from build123d import *

# Parameters (mm, degrees)
SKETCH_1_R           = 1.5
SKETCH_1_R_2         = 3
EXTRUDE_1_DEPTH      = 1
SKETCH_4_R           = 1.5
CUT_EXTRUDE_2_DEPTH  = 4
SKETCH_5_R           = 1.5
CUT_EXTRUDE_3_DEPTH  = 10
SKETCH_6_W           = 53
SKETCH_6_H           = 34
CUT_EXTRUDE_4_DEPTH  = 10
SKETCH_7_W           = 39
SKETCH_7_H           = 34
CUT_EXTRUDE_5_DEPTH  = 10
SKETCH_10_R          = 10
CUT_EXTRUDE_8_DEPTH  = 10
SKETCH_13_R          = 1.5
CUT_EXTRUDE_10_DEPTH = 1
FILLET_1_R           = 2
EXTRUDE_START        = -1
SKETCH_20_R          = 10
EXTRUDE_3_DEPTH      = 1
SKETCH_21_W          = 48
SKETCH_21_H          = 86
CUT_EXTRUDE_16_DEPTH = 10
FILLET_5_R           = 2


with BuildPart() as part:
    # 草图1 → 凸台-拉伸1 (new body)
    with BuildSketch(Plane.XY):
        Polygon((0, 0), (175, 0), (142.846096908, 120), (0, 120), align=None)
        with Locations((129, 25)):
            Circle(SKETCH_1_R, mode=Mode.SUBTRACT)
        with Locations((129, 5)):
            Circle(SKETCH_1_R, mode=Mode.SUBTRACT)
        with Locations((119, 15)):
            Circle(SKETCH_1_R_2, mode=Mode.SUBTRACT)
        with Locations((109, 5)):
            Circle(SKETCH_1_R, mode=Mode.SUBTRACT)
        with Locations((109, 25)):
            Circle(SKETCH_1_R, mode=Mode.SUBTRACT)
    extrude(amount=EXTRUDE_1_DEPTH)

    # 草图4 → 切除-拉伸2 (cut)
    with BuildSketch(Plane(origin=(0, 0, 0), x_dir=(-1, 0, 0), z_dir=(0, 0, -1))):
        with Locations((-22, 101)):
            Circle(SKETCH_4_R)
        with Locations((-22, 81)):
            Circle(SKETCH_4_R)
        with Locations((-22, 60)):
            Circle(SKETCH_4_R)
        with Locations((-22, 40)):
            Circle(SKETCH_4_R)
    extrude(amount=-CUT_EXTRUDE_2_DEPTH, mode=Mode.SUBTRACT)

    # 草图5 → 切除-拉伸3 (cut)
    with BuildSketch(Plane(origin=(0, 0, 0), x_dir=(-1, 0, 0), z_dir=(0, 0, -1))):
        with Locations((-136.2, 107)):
            Circle(SKETCH_5_R)
        with Locations((-124.2, 95)):
            Circle(SKETCH_5_R)
    extrude(amount=-CUT_EXTRUDE_3_DEPTH, mode=Mode.SUBTRACT)

    # 草图6 → 切除-拉伸4 (cut)
    with BuildSketch(Plane.XY.offset(1)):
        with Locations((26.5, 17)):
            Rectangle(SKETCH_6_W, SKETCH_6_H)
    extrude(amount=-CUT_EXTRUDE_4_DEPTH, mode=Mode.SUBTRACT)

    # 草图7 → 切除-拉伸5 (cut)
    with BuildSketch(Plane.XY.offset(1)):
        with Locations((72.5, 17)):
            Rectangle(SKETCH_7_W, SKETCH_7_H)
    extrude(amount=-CUT_EXTRUDE_5_DEPTH, mode=Mode.SUBTRACT)

    # 草图10 → 切除-拉伸8 (cut)
    with BuildSketch(Plane.XY.offset(1)):
        with Locations((37, 104)):
            Circle(SKETCH_10_R)
    extrude(amount=-CUT_EXTRUDE_8_DEPTH, mode=Mode.SUBTRACT)

    # 草图13 → 切除-拉伸10 (cut)
    with BuildSketch(Plane.XY.offset(1)):
        with Locations((121, 115)):
            Circle(SKETCH_13_R)
        with Locations((101, 115)):
            Circle(SKETCH_13_R)
        with Locations((80, 115)):
            Circle(SKETCH_13_R)
        with Locations((60, 115)):
            Circle(SKETCH_13_R)
        with Locations((45, 115)):
            Circle(SKETCH_13_R)
        with Locations((25, 115)):
            Circle(SKETCH_13_R)
    extrude(amount=-CUT_EXTRUDE_10_DEPTH, mode=Mode.SUBTRACT)

    # 圆角1
    fillet_1_edges = [part.edges().sort_by_distance(p)[0] for p in [
        (0, 34, 0.5),
        (0, 120, 0.5),
        (142.846096908, 120, 0.5),
        (175, 0, 0.5),
        (92, 34, 0.5),
        (92, 0, 0.5),
    ]]
    fillet(fillet_1_edges, radius=FILLET_1_R)

    # 草图20 → 凸台-拉伸3 (add)
    with BuildSketch(Plane(origin=(0, 0, 0), x_dir=(-1, 0, 0), z_dir=(0, 0, -1)).offset(EXTRUDE_START)):
        with Locations((-37, 104)):
            Circle(SKETCH_20_R)
    extrude(amount=EXTRUDE_3_DEPTH)

    # 草图21 → 切除-拉伸16 (cut)
    with BuildSketch(Plane(origin=(0, 0, 0), x_dir=(-1, 0, 0), z_dir=(0, 0, -1))):
        with Locations((-24, 77)):
            Rectangle(SKETCH_21_W, SKETCH_21_H)
    extrude(amount=-CUT_EXTRUDE_16_DEPTH, mode=Mode.SUBTRACT)

    # 圆角5
    fillet_5_edges = [part.edges().sort_by_distance(p)[0] for p in [
        (48, 34, 0.5),
        (48, 120, 0.5),
    ]]
    fillet(fillet_5_edges, radius=FILLET_5_R)


solid = part.part
Input: part model. Units: mm. Frame: model coordinates. Give positions to 0.01 mm unless a question says otherwise; leave off trailing zeros. Loops run counter-clockwise (first coordinate to the right, second up) from the corner with the lowest first, then second, coordinate; pieces in that order, holes last. Notation, with made-up numbers: (-9.75, 89) - (8.25, 89) arc R26 cw to (8.25, 121) - close; hole circle Ø3 at (-10, 68). An arc over 180 degrees is marked (long way). Use CSV: the item, a comma, the result in double quotes. Start each with the question number.
Item 1: Section D-D on y = 107. Return loops of the section in (x, z), then the cut area to 3 significant figures.
Item 2: Section B-B on z = 0.65. State how many separate pieces and enclosed holes the cut face has, then the cut area to 3 significant figures.
Item 3: Mould query, pull axis X, two halves, no side actions, for faces 1 (the flat face through (112, 61, 1)), 2 (the cylindrical face through (121.77, 13.85, 0.49)), 3 (the flat face through (159, 59.71, 0.49)). Classes: pulls with the +X half, pulls with the -X half, needs draft (parallel to the pull), parting line crosses it, or undercut.
Item 4: Section C-C on y = 25. Return loops of the section in (x, z), then the cut area to 3 significant figures.
Item 5: Section A-A on x = 101. Return loops of the section in (y, z).
Item 6: Line query: line 1 (Y direction, x = 129, z = 0.4); line 2 (Y direction, x = 124.2, z = 0.4); line 3 (X direction, y = 115, z = 0.85). Output: solid intervals per line, ascending.
Item 7: Contact query for a flat-ended pin moving along its axis: P1, Ø0.5, axis at x = 79.5, z = 0.5, coming from the -Y side. Output: stop coordinate, or through.
Ans:
1,outline,"(48, 0) - (134.7, 0) - (134.7, 1) - (48, 1) - close; (137.7, 0) - (146.33, 0) - (146.33, 1) - (137.7, 1) - close"
1,area,"95.3 mm2"
2,separate pieces,"1"
2,enclosed holes,"11"
2,area,"11,700 mm2"
3,face 1,"needs draft"
3,face 2,"undercut"
3,face 3,"pulls with the +X half"
4,outline,"(92, 0) - (107.5, 0) - (107.5, 1) - (92, 1) - close; (110.5, 0) - (127.5, 0) - (127.5, 1) - (110.5, 1) - close; (130.5, 0) - (168.3, 0) - (168.3, 1) - (130.5, 1) - close"
4,area,"70.3 mm2"
5,outline,"(0, 0) - (113.5, 0) - (113.5, 1) - (0, 1) - close; (116.5, 0) - (120, 0) - (120, 1) - (116.5, 1) - close"
6,line 1,"y = 0 to 3.5, 6.5 to 23.5, 26.5 to 120"
6,line 2,"y = 0 to 93.5, 96.5 to 120"
6,line 3,"x = 48 to 58.5, 61.5 to 78.5, 81.5 to 99.5, 102.5 to 119.5, 122.5 to 144.19"
7,P1,"stops at y = 34"
